For this review, use the dimensioned drawing (mm, ordinates from the lowest corner) and the shaded views. Give positions to 0.01 mm unless a question says otherwise; leave off trailing zeros. Write each loop counter-clockwise with the first axis right and the second up, starting at its lowest first coordinate (ties: lowest second). Pieces come first, ordered by that corner, then holes.
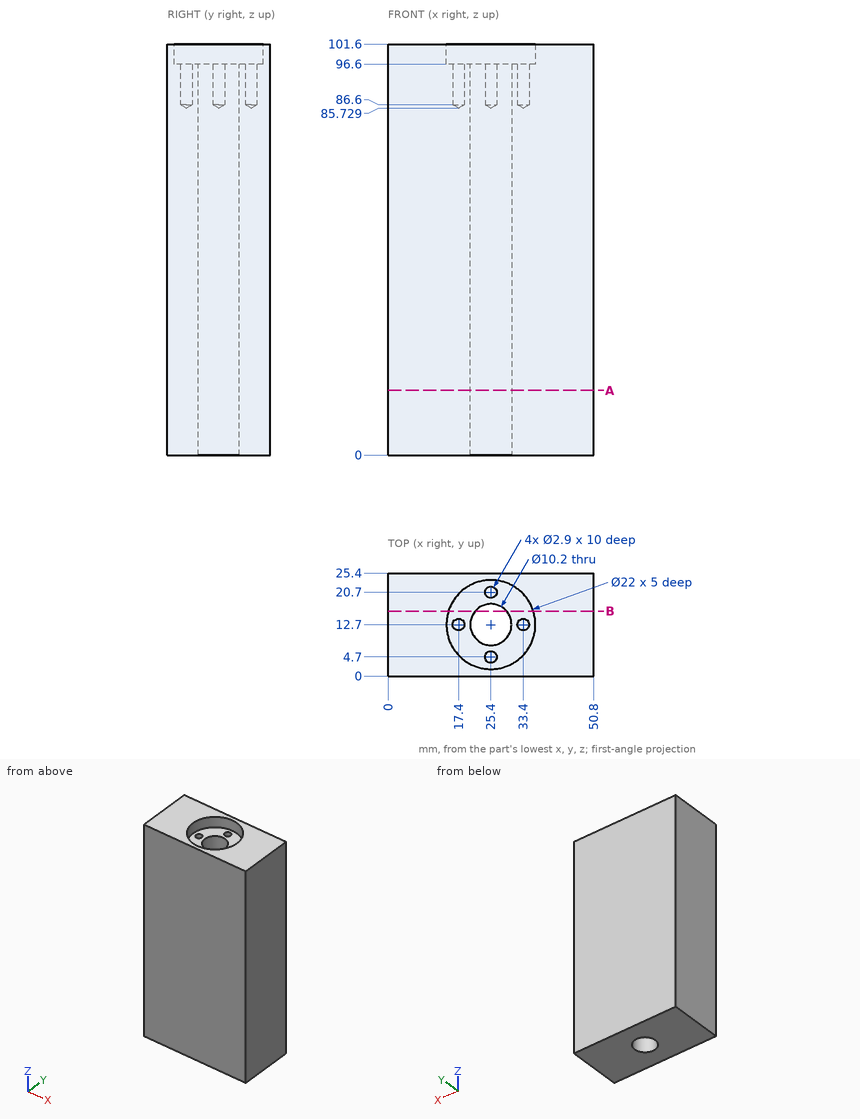
(1) We need section B-B (y = 16). Write out the cut boundary in (x, z), and give its area (4 significant figures).
(2) For L1, parallel to Y at x = 25.4, z = 24.5; L2, parallel to X at y = 13.25, z = 43.5; L3, parallel to Y at x = 28, z = 18, list the stretches that pass through material, from the lowest coordinate up.
(3) Clearance check with flat-ended pins moving along their axes: pin 1 Ø4 at (x, y) = (17.4, 12.7) entering from +Z; pin 2 Ø2.5 at (x, y) = (25.4, 4.7) entering from +Z. State where each tip first meets the part, or that it passes through.
(4) We need section A-A (z = 16). Write out the cut boundary in (x, y).
The answers:
1. outline: (0, 0) - (21.51, 0) - (21.51, 96.6) - (14.91, 96.6) - (14.91, 101.6) - (0, 101.6) - close; (29.29, 0) - (50.8, 0) - (50.8, 101.6) - (35.89, 101.6) - (35.89, 96.6) - (29.29, 96.6) - close
1. area: 4,305 mm2
2. L1: y = 0 to 7.6, 17.8 to 25.4
2. L2: x = 0 to 20.33, 30.47 to 50.8
2. L3: y = 0 to 8.31, 17.09 to 25.4
3. pin 1: stops at z = 96.6
3. pin 2: stops at z = 86.48
4. outline: (0, 0) - (50.8, 0) - (50.8, 25.4) - (0, 25.4) - close; hole circle Ø10.2 at (25.4, 12.7)
